Check sheet for the modelled part. Datum: model origin and axes. Units: mm. A direction names the side the tool comes from. Round coordinates to 2 decimals unless told otherwise and drop trailing zeros. Write each loop counter-clockwise with the first axis right and the second up, starting at its lowest first coordinate (ties: lowest second). Pieces come first, ordered by that corner, then holes. Notation, with made-up numbers: M 25,-14.75 L 65,-14.75 A19 cw 65,-9.75 Z; hole C 45.5,62.5 d9. An arc over 180 degrees is marked long. Put each result on its own line as item: value.
```python
from build123d import *

# Parameters (mm, degrees)
F1_DEPTH = 10
F4_SIZE  = 3
F5_R     = 8
F6_R     = 5


with BuildPart() as f1:
    # F0 (on Front) → F1 (new body, symmetric)
    with BuildSketch(Plane.XZ):
        with BuildLine():
            ThreePointArc((-50, 22), (-28, 0), (-50, -22))
            Line((-50, -22), (-50, -28))
            ThreePointArc((-50, -28), (-42.7848180337, -27.0544109009), (-36.0569644542, -24.2815106566))
            ThreePointArc((-36.0569644542, -24.2815106566), (-25.7677384951, -14.0284533131), (-22, 0))
            ThreePointArc((-22, 0), (0, 22), (22, 0))
            ThreePointArc((22, 0), (25.7677384951, -14.0284533131), (36.0569644542, -24.2815106566))
            ThreePointArc((36.0569644542, -24.2815106566), (42.7848180337, -27.0544109009), (50, -28))
            Line((50, -28), (50, -22))
            ThreePointArc((50, -22), (28, 0), (50, 22))
            Line((50, 22), (50, 28))
            ThreePointArc((50, 28), (35.3212154107, 23.8439359792), (25, 12.6095202129))
            ThreePointArc((25, 12.6095202129), (0, 28), (-25, 12.6095202129))
            ThreePointArc((-25, 12.6095202129), (-35.3212154107, 23.8439359792), (-50, 28))
            Line((-50, 28), (-50, 22))
        make_face()
    extrude(amount=F1_DEPTH, both=True)

    # F2 (on Front) → F3 (revolve, cut)
    with BuildSketch(Plane.XZ):
        Polygon((0, 31.6328920043), (-2, 31.6328920043), (-2, 26.3877877519), (-8.5819354281, 19.8058523238), (0, 19.8058523238), align=None)
    revolve(axis=Axis((0, 0, 16.2401215483), (0, 0, 1)), mode=Mode.SUBTRACT)

    # F4
    f4_edges = [f1.edges().sort_by_distance(p)[0] for p in [
        (-28, 10, 0),
        (-28, -10, 0),
        (28, 10, 0),
        (28, -10, 0),
    ]]
    chamfer(f4_edges, length=F4_SIZE)

    # F5
    f5_edges = [f1.edges().sort_by_distance(p)[0] for p in [
        (-28, 7, 0),
        (-28, -7, 0),
        (28, 7, 0),
        (28, -7, 0),
    ]]
    fillet(f5_edges, radius=F5_R)

    # F6
    f6_edges = [f1.edges().sort_by_distance(p)[0] for p in [
        (25, 0, 12.60952),
        (-25, 0, 12.60952),
    ]]
    fillet(f6_edges, radius=F6_R)


solid = f1.part
```
1. Depth check by flat-ended pin: pin 1 Ø1.5 at (y, z) = (-6.5, -8.5) entering from -X; pin 2 Ø2 at (y, z) = (2.5, 18.5) entering from -X; pin 3 Ø1.5 at (x, y) = (30, -7) entering from -Z. Enter the tip coordinate at first touch or a pass-through.
Computed values:
pin 1: stops at x = -29.58
pin 2: stops at x = -39.81
pin 3: stops at z = -20.33
2. Access from +Z, -Z, +X, -X, +Y, -Y to the whole of each face (thin tool, end or side, straight path). Record for faces 5 (the flat face through (50, 0, -25)), 6 (the cylindrical face through (38.486, -0.14, 25.523)), 7 (the cylindrical face through (-30.42, -0.14, -20.015)).
Computed values:
face 5: +Z, -Z, +X, +Y, -Y
face 6: +Z, +Y, -Y
face 7: -Z, +Y, -Y
3. Scan lines: probe 1 along Y at (x, z) = (0, 26.95); probe 2 along X at (y, z) = (8, -5.5); probe 3 along Z at (x, y) = (-33, -7). Record each from-to range of solid material in increasing order.
Computed values:
probe 1: y = -10 to -2, 2 to 10
probe 2: x = -27.4 to -22.55, 22.55 to 27.4
probe 3: z = -22.25 to -15.07, 15.07 to 22.25
4. Release check for a two-part mould opening along Z. For faces 1 (the cylindrical face through (-28, 0, 0)), 2 (the flat face through (-50, 0, -25)), 3 (the cylindrical face through (0.3, -2.4, 28)), 4 (the cylindrical face through (29.985, -0.14, -19.58)) record: +Z half, -Z half, draft (parallel to the pull), parting line (faces both ways), or undercut.
Computed values:
face 1: undercut
face 2: draft
face 3: +Z half
face 4: -Z half
5. Cross-section at A-A (x = 0). Enter the section's corners in (y, z), then the cut area to 3 significant figures.
Computed values:
outline: M -10,22 L -6.39,22 L -2,26.39 L -2,28 L -10,28 Z; M 2,26.39 L 6.39,22 L 10,22 L 10,28 L 2,28 Z
area: 76.7 mm2
